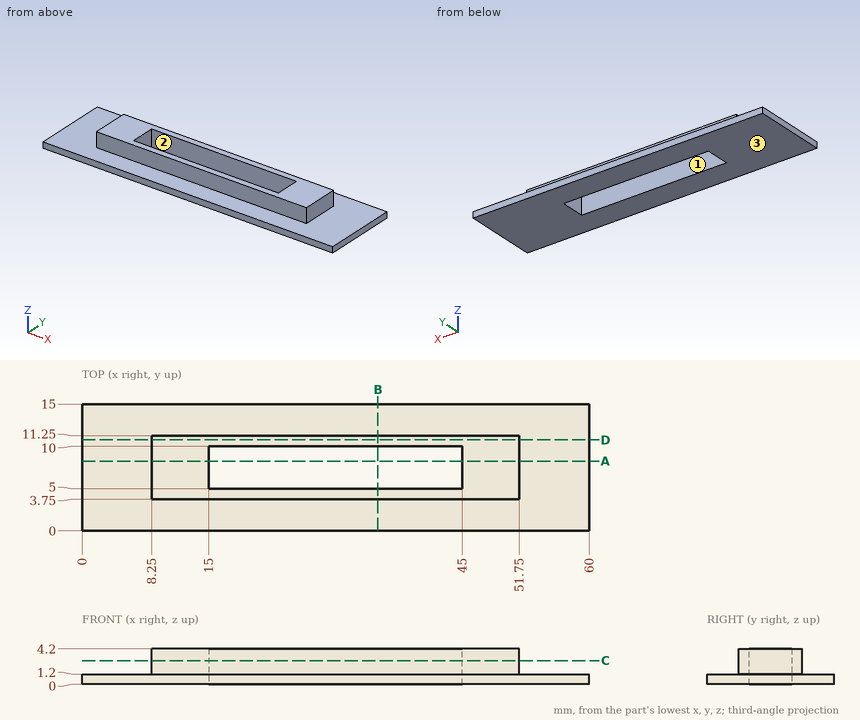
Study the drawing (mm; zero at the part's minimum x, y, z) and answer. Give positions to 0.01 mm unless a question says otherwise; leave off trailing zeros. Write each loop counter-clockwise with the first axis right and the second up, starting at its lowest first coordinate (ties: lowest second). Pieces come first, ordered by that corner, then holes.
(1) Flat-ended cylindrical pins translate along their axes: pin 1 Ø1.5 at (y, z) = (8, 2.5) entering from -X; pin 2 Ø5 at (x, y) = (28.5, 3.5) entering from +Z; pin 3 Ø0.9 at (y, z) = (9.5, 3) entering from +X. Find the tip coordinate at first contact, or state that the pin passes through.
Final values:
pin 1: stops at x = 8.25
pin 2: stops at z = 4.2
pin 3: stops at x = 51.75
(2) The mould has two halves that part along Y. Classify the marked faces 1, 2 and 3: pulls with the +Y half, pulls with the -Y half, needs draft (parallel to the pull), parting line crosses it, or undercut.
Final values:
face 1: undercut
face 2: undercut
face 3: needs draft
(3) The part is cut by section A-A on y = 8.25. Write down the section's boundary in (x, z), plus the area to 3 significant figures.
Final values:
outline: (0, 0) - (15, 0) - (15, 4.2) - (8.25, 4.2) - (8.25, 1.2) - (0, 1.2) - close; (45, 0) - (60, 0) - (60, 1.2) - (51.75, 1.2) - (51.75, 4.2) - (45, 4.2) - close
area: 76.5 mm2
(4) The part is cut by section B-B on x = 35. Write down the section's boundary in (y, z), plus the area to 3 significant figures.
Final values:
outline: (0, 0) - (5, 0) - (5, 4.2) - (3.75, 4.2) - (3.75, 1.2) - (0, 1.2) - close; (10, 0) - (15, 0) - (15, 1.2) - (11.25, 1.2) - (11.25, 4.2) - (10, 4.2) - close
area: 19.5 mm2
(5) The part is cut by section D-D on y = 10.75. Write down the section's boundary in (x, z).
Final values:
outline: (0, 0) - (60, 0) - (60, 1.2) - (51.75, 1.2) - (51.75, 4.2) - (8.25, 4.2) - (8.25, 1.2) - (0, 1.2) - close
(6) The part is cut by section C-C on z = 2.8. Write down the section's boundary in (x, y), plus the area to 3 significant figures.
Final values:
outline: (8.25, 3.75) - (51.75, 3.75) - (51.75, 11.25) - (8.25, 11.25) - close; hole (15, 5) - (45, 5) - (45, 10) - (15, 10) - close
area: 176 mm2
(7) Straight lines are drawn through the part: line 1 (X direction, y = 8.5, z = 1.8); line 2 (Y direction, x = 15.5, z = 2.15); line 3 (X direction, y = 6.75, z = 0.35). For each, find the intervals that lie inside material, in ascending order.
Final values:
line 1: x = 8.25 to 15, 45 to 51.75
line 2: y = 3.75 to 5, 10 to 11.25
line 3: x = 0 to 15, 45 to 60
